Print and shaded views of the part. All mm, measured from the part's lowest x, y and z. A direction names the side the tool comes from. Give positions to 0.01 mm unless a question says otherwise; leave off trailing zeros. Loops run counter-clockwise (first coordinate to the right, second up) from the corner with the lowest first, then second, coordinate; pieces in that order, holes last. Notation, with made-up numbers: M -32,63 L -17,63 A12 ccw -17,79 Z; hole C 20,16 d3. An arc over 180 degrees is marked long. Put each result on its own line as item: value. Start each with the question number.
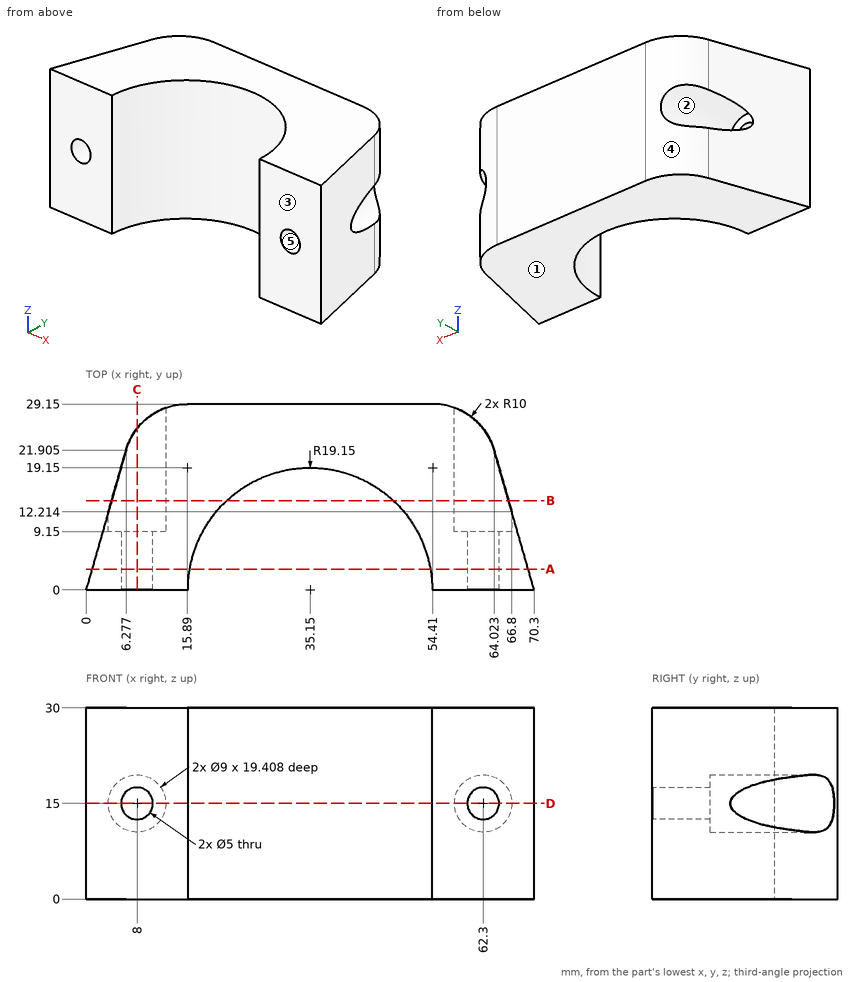
1) Band-saw the part on C-C on x = 8. Give the cut face in (y, z), then the cut area to 3 significant figures.
2) Mould opens along X. For the marked faces 3, 4 and 5 say: +X half, -X half, draft (parallel to the pull), parting line (faces both ways), or undercut.
3) Band-saw the part on A-A on y = 3.25. Give the cut face in (x, z).
4) Pin check, flat tips, straight feed: pin 1 Ø4 at (x, z) = (12.5, 10) entering from +Y; pin 2 Ø11.5 at (x, z) = (62.3, 15) entering from +Y; pin 3 Ø1 at (x, z) = (63, 7.5) entering from +Y. Stop position of each tip, or through.
5) Wall check: L1, parallel to Z at x = 62.3, y = 14; L2, parallel to Z at x = 8, y = 2.25; L3, parallel to X at y = 11, z = 12.5 (1 decimal). Give the ranges that are in metal, low to high.
6) Which spindle directions (+Z, -Z, +X, -X, +Y, -Y) get a long thin tool onto all of the face, cutting with end or side? Do the marked faces 1 and 2. Say none if no direction does.
7) Band-saw the part on D-D on z = 15. State how many separate pieces and enclosed holes the cut face has, then the cut area to 3 significant figures.
8) Band-saw the part on B-B on y = 14. Give the cut face in (x, z).
Evaluation:
1. outline: M 0,0 L 25.29,0 L 25.29,10.5 L 9.15,10.5 L 9.15,12.5 L 0,12.5 Z; M 0,17.5 L 9.15,17.5 L 9.15,19.5 L 25.29,19.5 L 25.29,30 L 0,30 Z
1. area: 568 mm2
2. face 3: draft
2. face 4: -X half
2. face 5: undercut
3. outline: M 0.93,0 L 16.28,0 L 16.28,30 L 0.93,30 Z; M 54.02,0 L 69.37,0 L 69.37,30 L 54.02,30 Z; hole C 8,15 d5; hole C 62.3,15 d5
4. pin 1: y = 29.05
4. pin 2: y = 28.92
4. pin 3: y = 25.03
5. L1: 0 to 10.5, 19.5 to 30
5. L2: 0 to 12.5, 17.5 to 30
5. L3: 3.2 to 4.3, 11.7 to 19.5, 50.8 to 58.6, 66 to 67.1
6. face 1: -Z, +X, -X, +Y, -Y
6. face 2: +Y
7. separate pieces: 3
7. enclosed holes: 0
7. area: 859 mm2
8. outline: M 4.01,0 L 22.08,0 L 22.08,30 L 4.01,30 L 4.01,17.08 A4.5 cw long 4.01,12.92 Z; M 48.22,0 L 66.29,0 L 66.29,12.92 A4.5 cw long 66.29,17.08 L 66.29,30 L 48.22,30 Z
